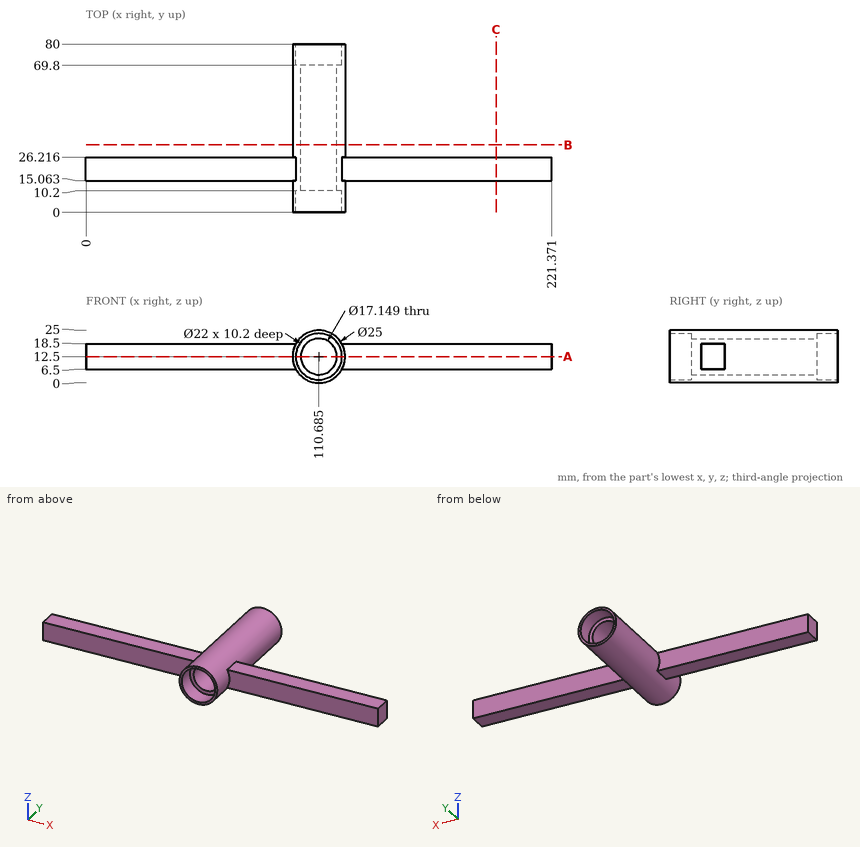
Input: dimensioned drawing with shaded views. Units: mm. Origin: part minimum x, y, z. Coordinates: 2 decimals unless noted, no trailing zeros. Loops run counter-clockwise (first coordinate to the right, second up) from the corner with the lowest first, then second, coordinate; pieces in that order, holes last. Notation, with made-up numbers: M -5.75,13.5 L 32.25,13.5 A36 cw 32.25,52.5 Z; hole C 5,0 d6. An arc over 180 degrees is marked long. Use a Markdown table: item, result. Add a question column.
1) Section B-B, the plane y = 32. Return the cut outline in (x, z) (1 decimal), plus the area to 3 significant figures.
2) Section C-C, the plane x = 195. Return the cut outline in (y, z), plus the area to 3 significant figures.
3) Line query: L1, parallel to X at y = 70, z = 11.5 (1 decimal); L2, parallel to Y at x = 178, z = 18; L3, parallel to X at y = 74.5, z = 17 (1 decimal). Output: solid intervals per line, ascending. Write a range as from..to.
4) Pin query (flat end, axial travel): P1, Ø12.5, axis at x = 45.5, y = 18.5, coming from the -Z side; P2, Ø4, axis at x = 79.5, y = 13.5, coming from the +Z side; P3, Ø10, axis at x = 36.5, z = 7, coming from the +Y side. Return the tip coordinate at first contact, or that it passes through.
5) Section A-A, the plane z = 12.5. Return the cut outline in (x, y) (1 decimal).
Answer below:
| question | item | result |
|---|---|---|
| 1 | outline | C 110.7,12.5 d25; hole C 110.7,12.5 d17.1 |
| 1 | area | 260 mm2 |
| 2 | outline | M 15.06,6.5 L 26.22,6.5 L 26.22,18.5 L 15.06,18.5 Z |
| 2 | area | 134 mm2 |
| 3 | L1 | 98.2..99.7, 121.6..123.1 |
| 3 | L2 | 15.06..26.22 |
| 3 | L3 | 99..100.6, 120.7..122.3 |
| 4 | P1 | z = 6.5 |
| 4 | P2 | z = 18.5 |
| 4 | P3 | y = 26.22 |
| 5 | outline | M 0,15.1 L 98.2,15.1 L 98.2,0 L 99.7,0 L 99.7,10.2 L 102.1,10.2 L 102.1,69.8 L 99.7,69.8 L 99.7,80 L 98.2,80 L 98.2,26.2 L 0,26.2 Z; M 119.3,10.2 L 121.7,10.2 L 121.7,0 L 123.2,0 L 123.2,15.1 L 221.4,15.1 L 221.4,26.2 L 123.2,26.2 L 123.2,80 L 121.7,80 L 121.7,69.8 L 119.3,69.8 Z |
